Autodesk Inventor part; units mm, degrees
ref_plane "YZ Plane" through (0, 0, 0) normal (1, 0, 0) x (0, 1, 0)
ref_plane "XZ Plane" through (0, 0, 0) normal (0, 1, 0) x (-1, 0, 0)
ref_plane "XY Plane" through (0, 0, 0) normal (0, 0, 1) x (1, 0, 0)
sketch "Sketch1" plane through (0, 0, 0) normal (0, 1, 0) x (-1, 0, 0)
  arc A0 (-31.8654, -4.9656) -> (31.8654, -4.9656) centre (0, 0) ccw
  arc A1 (-38.9338, 4.9718) -> (38.9338, 4.9718) centre (0, 0) ccw
  line L0 (39.25, 0) -> (-39.25, 0)
  line L1 (35.3996, 0) -> (35.3996, 2)
  line L2 (35.3996, 2) -> (35.3996, -2)
  line L3 (36.0047, -4.9656) -> (31.8654, -4.9656)
  line L4 (34.7945, 4.9718) -> (38.9338, 4.9718)
  line L5 (35.3996, 2) -> (34.2752, 2)
  line L6 (34.2752, 2) -> (34.2752, 4.9718)
  line L7 (34.2752, 4.9718) -> (34.7945, 4.9718)
  line L8 (36.0047, -4.9656) -> (36.5241, -4.9656)
  line L9 (36.5241, -4.9656) -> (36.5241, -2)
  line L10 (36.5241, -2) -> (35.3996, -2)
  line L11 (0, 0) -> (0, -17)
  line L12 (-35.3996, 0) -> (-35.3996, 2)
  line L13 (-35.3996, 2) -> (-35.3996, -2)
  line L14 (-36.0047, -4.9656) -> (-31.8654, -4.9656)
  line L15 (-34.7945, 4.9718) -> (-38.9338, 4.9718)
  line L16 (-35.3996, 2) -> (-34.2752, 2)
  line L17 (-34.2752, 2) -> (-34.2752, 4.9718)
  line L18 (-34.2752, 4.9718) -> (-34.7945, 4.9718)
  line L19 (-36.0047, -4.9656) -> (-36.5241, -4.9656)
  line L20 (-36.5241, -4.9656) -> (-36.5241, -2)
  line L21 (-36.5241, -2) -> (-35.3996, -2)
  arc A2 (-38.9338, 4.9718) -> (38.9338, 4.9718) centre (0, 0) ccw
  arc A3 (-36.5232, 4.9718) -> (36.5232, 4.9718) centre (0, 0) ccw
  line L22 (-36.5232, 4.9718) -> (-38.9338, 4.9718)
  line L23 (38.9338, 4.9718) -> (36.5232, 4.9718)
  dimension "d0" = 64.5
  dimension "d1" = 7
extrude "Extrusion1" add sketch "Sketch1" along normal blind 105 contours A0 L3 L8 A3 L19 L14 | A3 L0 L13 L21 L20 | A3 L0 A1 | L9 L10 L2 L0 A3 | A3 L15 L18 L17 L16 L12 L0 | L0 A1 L15 A3 | A3 L4 A1 L0 | L0 L1 L5 L6 L7 L4 A3
chamfer "Chamfer1" distance 0.5 angle 45 6 edges at (-34.2752, 52.5, 2) (-35.3996, 52.5, -2) (-34.2752, 52.5, 4.9718) (35.3996, 52.5, -2) (34.2752, 52.5, 2) (34.2752, 52.5, 4.9718)
extrude "Extrusion2" add sketch "Sketch1" against normal blind 5 contours A3 L0 A1 | L0 A1 L15 A3 | A3 L4 A1 L0
properties part number "cyl outer"
Can you work these out from the model? Positions are in its coordinate system, mm. A direction names the side the tool comes from. Round coordinates to 2 decimals unless told otherwise and drop trailing zeros. Order: outer loops, then holes, each group sorted by start corner. A loop starts at its lowest first (then second) coordinate and runs counter-clockwise, first axis right, second up.
(1) If we section it at A-A (z = 0): Please give me the cut outline in (x, y).
Results are:
outline: (-39.25, -5) - (-36.86, -5) - (-36.86, 0) - (-35.4, 0) - (-35.4, 105) - (-39.25, 105) - close; (35.4, 0) - (36.86, 0) - (36.86, -5) - (39.25, -5) - (39.25, 105) - (35.4, 105) - close
(2) If we section it at B-B (y = 9.5): Please give me the cut outline in (x, z).
Results are:
outline: (-38.93, 4.97) arc R39.25 ccw (long way) to (38.93, 4.97) - (34.78, 4.97) - (34.28, 4.47) - (34.28, 2.5) - (34.78, 2) - (35.4, 2) - (35.4, -1.5) - (35.9, -2) - (36.52, -2) - (36.52, -4.97) - (31.87, -4.97) arc R32.25 cw to (-31.87, -4.97) - (-36.52, -4.97) - (-36.52, -2) - (-35.9, -2) - (-35.4, -1.5) - (-35.4, 2) - (-34.78, 2) - (-34.28, 2.5) - (-34.28, 4.47) - (-34.78, 4.97) - close
(3) If we section it at C-C (z = -19): Please give me the cut outline in (x, y), plus the area to 3 significant figures.
Results are:
outline: (-34.34, -5) - (-31.59, -5) - (-31.59, 0) - (-26.06, 0) - (-26.06, 105) - (-34.34, 105) - close; (26.06, 0) - (31.59, 0) - (31.59, -5) - (34.34, -5) - (34.34, 105) - (26.06, 105) - close
area: 1,770 mm2
(4) If we section it at D-D (x = 0): Please give me the cut outline in (y, z), plus the area to 3 significant figures.
Results are:
outline: (-5, -39.25) - (105, -39.25) - (105, -32.25) - (0, -32.25) - (0, -36.86) - (-5, -36.86) - close
area: 747 mm2
(5) We'd pull the mould along Z, two halves only. Please class faces 1 (the face through (37, 49, 4.972)), 2 (the face through (6, -5, -37)), 3 (the face through (36.524, 52, -4)): +Z half, -Z half, draft (parallel to the pull), parting line (faces both ways), or undercut.
Results are:
face 1: +Z half
face 2: draft
face 3: undercut
(6) On a 3-axis mill with a long thin cutter (end or side, diameter ignored), from which of +Z, -Z, +X, -X, +Y, -Y can I reach the whole of each face in a straight line? I mean faces 4 (the face through (0.88, -2.46, -36.85)), 5 (the face through (-34, 52, -4.966)), 6 (the face through (0, 0, -33)). Say none if no direction works.
Results are:
face 4: -Y
face 5: +Y, -Y
face 6: +Z, -Y
(7) I'm going to push flat-ended pins straight in: pin 1 (8 mm diameter, centred on y = 84, z = -13.5, fed in from +X); pin 2 (0.6 mm diameter, centred on y = 52.5, z = 3, fed in from -X); pin 3 (1.5 mm diameter, centred on y = 60.5, z = -32, fed in from +X). Where does each tip first touch, or does it pass through?
Results are:
pin 1: stops at x = 38.08
pin 2: stops at x = -39.16
pin 3: stops at x = 23.75
(8) If I drill on L1, parallel to X at y = -1.3, z = 0; L2, parallel to X at y = 57.5, z = 1.5; L3, parallel to Y at x = 36.5, z = 0.5, over which ranges is the centre line in solid material (lowest first)?
Results are:
L1: x = -39.25 to -36.86, 36.86 to 39.25
L2: x = -39.22 to -35.4, 35.4 to 39.22
L3: y = 0 to 105
